Input: part model. Units: mm. Frame: model coordinates. Face numbers are marked on the shaded views. A direction names the side the tool comes from. Round coordinates to 2 decimals unless told otherwise and drop trailing zeros. Order: outer loops, then holes, each group sorted by start corner. A loop starts at its lowest first (then second) coordinate and runs counter-clockwise, first axis right, second up. Notation, with made-up numbers: M 58,66.5 L 94,66.5 A12 ccw 94,71.5 Z; hole C 74,6 d5. An arc over 180 degrees is marked long. One line per question, with ' | ' between items.
```python
from build123d import *

# Parameters (mm, degrees)
SKETCH_2_W                  = 36.9
SKETCH_2_H                  = 60.6
SKETCH_2_W_2                = 33.7
SKETCH_2_H_2                = 57.4
SKETCH_2_W_3                = 35.4
SKETCH_2_H_3                = 59.1
SKETCH_2_R                  = 3.75
SKETCH_2_R_2                = 2.25
SKETCH_2_R_3                = 0.75
EXTRUDE_1_DEPTH             = 1.5
EXTRUDE_START               = 1.5
SKETCH_2_20_W               = 36.9
SKETCH_2_20_H               = 60.6
SKETCH_2_20_W_2             = 35.4
SKETCH_2_20_H_2             = 59.1
SKETCH_2_20_W_3             = 33.7
SKETCH_2_20_H_3             = 57.4
EXTRUDE_9_DEPTH             = 12
CUT_EXTRUDE_START           = 13.5
SKETCH_2_21_W               = 35.4
SKETCH_2_21_H               = 59.1
SKETCH_2_21_W_2             = 33.7
SKETCH_2_21_H_2             = 57.4
CUT_EXTRUDE_3_DEPTH         = 1.5
EXTRUDE_START_2             = 13.5
SKETCH_2_23_R               = 3
SKETCH_2_23_R_2             = 1.6
EXTRUDE_10_DEPTH            = 10
FILLET_2_R                  = 3.5
HOLE_WIZARD_M32_D           = 3.4
HOLE_WIZARD_M32_CSINK_D     = 6.72
HOLE_WIZARD_M32_CSINK_ANGLE = 90
SKETCH_12_W                 = 1.6
SKETCH_12_H                 = 15.6
SKETCH_12_H_2               = 15.8
SKETCH_12_H_3               = 12.5
CUT_EXTRUDE_4_DEPTH         = 1.65
SKETCH_13_W                 = 3
SKETCH_13_H                 = 10
SKETCH_13_H_2               = 7
SKETCH_13_W_2               = 10
SKETCH_13_H_3               = 3
EXTRUDE_11_DEPTH            = 16.2


with BuildPart() as part:
    # Эскиз2 → Бобышка-Вытянуть1 (new body)
    # profile 1 of 15: a face of its own
    with BuildSketch(Plane(origin=(0, 0, 0), x_dir=(1, 0, 0), z_dir=(0, 1, 0))):
        with Locations((16.65, 28.5)):
            Rectangle(SKETCH_2_W, SKETCH_2_H)
        with Locations((16.65, 28.5)):
            Rectangle(SKETCH_2_W_2, SKETCH_2_H_2, mode=Mode.SUBTRACT)
    # profile 2 of 15: a face of its own
    with BuildSketch(Plane(origin=(0, 0, 0), x_dir=(1, 0, 0), z_dir=(0, 1, 0))):
        with Locations((16.65, 28.5)):
            Rectangle(SKETCH_2_W_3, SKETCH_2_H_3)
        with Locations((16.65, 28.5)):
            Rectangle(SKETCH_2_W_2, SKETCH_2_H_2, mode=Mode.SUBTRACT)
    # profile 3 of 15: a face of its own
    with BuildSketch(Plane(origin=(0, 0, 0), x_dir=(1, 0, 0), z_dir=(0, 1, 0))):
        with BuildLine():
            Line((-0.2, 57.2), (-0.2, -0.2))
            Line((-0.2, -0.2), (33.5, -0.2))
            Line((33.5, -0.2), (33.5, 10.050490243))
            ThreePointArc((33.5, 10.050490243), (27, 12.6), (33.5, 15.149509757))
            Line((33.5, 15.149509757), (33.5, 57.2))
            Line((33.5, 57.2), (-0.2, 57.2))
        make_face()
        with Locations((5.1, 19.73)):
            Circle(SKETCH_2_R, mode=Mode.SUBTRACT)
        with Locations((5.1, 41.13)):
            Circle(SKETCH_2_R, mode=Mode.SUBTRACT)
        with Locations((23.55, 45)):
            Circle(SKETCH_2_R, mode=Mode.SUBTRACT)
    # profile 4 of 15: a face of its own
    with BuildSketch(Plane(origin=(0, 0, 0), x_dir=(1, 0, 0), z_dir=(0, 1, 0))):
        with Locations((23.55, 45)):
            Circle(SKETCH_2_R)
        with Locations((23.55, 45)):
            Circle(SKETCH_2_R_2, mode=Mode.SUBTRACT)
    # profile 5 of 15: a face of its own
    with BuildSketch(Plane(origin=(0, 0, 0), x_dir=(1, 0, 0), z_dir=(0, 1, 0))):
        with Locations((23.55, 45)):
            Circle(SKETCH_2_R_2)
        with Locations((23.55, 45)):
            Circle(SKETCH_2_R_3, mode=Mode.SUBTRACT)
    # profile 6 of 15: a face of its own
    with BuildSketch(Plane(origin=(0, 0, 0), x_dir=(1, 0, 0), z_dir=(0, 1, 0))):
        with Locations((23.55, 45)):
            Circle(SKETCH_2_R_3)
    # profile 7 of 15: a face of its own
    with BuildSketch(Plane(origin=(0, 0, 0), x_dir=(1, 0, 0), z_dir=(0, 1, 0))):
        with Locations((5.1, 41.13)):
            Circle(SKETCH_2_R)
        with Locations((5.1, 41.13)):
            Circle(SKETCH_2_R_2, mode=Mode.SUBTRACT)
    # profile 8 of 15: a face of its own
    with BuildSketch(Plane(origin=(0, 0, 0), x_dir=(1, 0, 0), z_dir=(0, 1, 0))):
        with Locations((5.1, 41.13)):
            Circle(SKETCH_2_R_2)
        with Locations((5.1, 41.13)):
            Circle(SKETCH_2_R_3, mode=Mode.SUBTRACT)
    # profile 9 of 15: a face of its own
    with BuildSketch(Plane(origin=(0, 0, 0), x_dir=(1, 0, 0), z_dir=(0, 1, 0))):
        with Locations((5.1, 41.13)):
            Circle(SKETCH_2_R_3)
    # profile 10 of 15: a face of its own
    with BuildSketch(Plane(origin=(0, 0, 0), x_dir=(1, 0, 0), z_dir=(0, 1, 0))):
        with Locations((5.1, 19.73)):
            Circle(SKETCH_2_R)
        with Locations((5.1, 19.73)):
            Circle(SKETCH_2_R_2, mode=Mode.SUBTRACT)
    # profile 11 of 15: a face of its own
    with BuildSketch(Plane(origin=(0, 0, 0), x_dir=(1, 0, 0), z_dir=(0, 1, 0))):
        with Locations((5.1, 19.73)):
            Circle(SKETCH_2_R_2)
        with Locations((5.1, 19.73)):
            Circle(SKETCH_2_R_3, mode=Mode.SUBTRACT)
    # profile 12 of 15: a face of its own
    with BuildSketch(Plane(origin=(0, 0, 0), x_dir=(1, 0, 0), z_dir=(0, 1, 0))):
        with Locations((5.1, 19.73)):
            Circle(SKETCH_2_R_3)
    # profile 13 of 15: a face of its own
    with BuildSketch(Plane(origin=(0, 0, 0), x_dir=(1, 0, 0), z_dir=(0, 1, 0))):
        with BuildLine():
            ThreePointArc((33.5, 15.149509757), (27, 12.6), (33.5, 10.050490243))
            Line((33.5, 10.050490243), (33.5, 15.149509757))
        make_face()
        with Locations((30.75, 12.6)):
            Circle(SKETCH_2_R_2, mode=Mode.SUBTRACT)
    # profile 14 of 15: a face of its own
    with BuildSketch(Plane(origin=(0, 0, 0), x_dir=(1, 0, 0), z_dir=(0, 1, 0))):
        with Locations((30.75, 12.6)):
            Circle(SKETCH_2_R_2)
        with Locations((30.75, 12.6)):
            Circle(SKETCH_2_R_3, mode=Mode.SUBTRACT)
    # profile 15 of 15: a face of its own
    with BuildSketch(Plane(origin=(0, 0, 0), x_dir=(1, 0, 0), z_dir=(0, 1, 0))):
        with Locations((30.75, 12.6)):
            Circle(SKETCH_2_R_3)
    extrude(amount=EXTRUDE_1_DEPTH)

    # Эскиз2<20> → Бобышка-Вытянуть9 (add)
    # profile 1 of 2: a face of its own
    with BuildSketch(Plane(origin=(0, 0, 0), x_dir=(1, 0, 0), z_dir=(0, 1, 0)).offset(EXTRUDE_START)):
        with Locations((16.65, 28.5)):
            Rectangle(SKETCH_2_20_W, SKETCH_2_20_H)
        with Locations((16.65, 28.5)):
            Rectangle(SKETCH_2_20_W_2, SKETCH_2_20_H_2, mode=Mode.SUBTRACT)
    # profile 2 of 2: a face of its own
    with BuildSketch(Plane(origin=(0, 0, 0), x_dir=(1, 0, 0), z_dir=(0, 1, 0)).offset(EXTRUDE_START)):
        with Locations((16.65, 28.5)):
            Rectangle(SKETCH_2_20_W_2, SKETCH_2_20_H_2)
        with Locations((16.65, 28.5)):
            Rectangle(SKETCH_2_20_W_3, SKETCH_2_20_H_3, mode=Mode.SUBTRACT)
    extrude(amount=EXTRUDE_9_DEPTH)

    # Эскиз2<21> → Вырез-Вытянуть3 (cut)
    with BuildSketch(Plane(origin=(0, 0, 0), x_dir=(1, 0, 0), z_dir=(0, 1, 0)).offset(CUT_EXTRUDE_START)):
        with Locations((16.65, 28.5)):
            Rectangle(SKETCH_2_21_W, SKETCH_2_21_H)
        with Locations((16.65, 28.5)):
            Rectangle(SKETCH_2_21_W_2, SKETCH_2_21_H_2, mode=Mode.SUBTRACT)
    extrude(amount=-CUT_EXTRUDE_3_DEPTH, mode=Mode.SUBTRACT)

    # Эскиз2<23> → Бобышка-Вытянуть10 (add)
    # profile 1 of 4: a face of its own
    with BuildSketch(Plane(origin=(0, 0, 0), x_dir=(1, 0, 0), z_dir=(0, 1, 0)).offset(EXTRUDE_START_2)):
        with BuildLine():
            ThreePointArc((7.877165354, 60.877946056), (6.171513422, 59.351502874), (3.95, 58.8))
            Line((3.95, 58.8), (29.35, 58.8))
            ThreePointArc((29.35, 58.8), (27.128486578, 59.351502874), (25.422834646, 60.877946056))
            Line((25.422834646, 60.877946056), (21.403937008, 66.784591616))
            ThreePointArc((21.403937008, 66.784591616), (19.339200458, 68.632391258), (16.65, 69.3))
            ThreePointArc((16.65, 69.3), (13.960799542, 68.632391258), (11.896062992, 66.784591616))
            Line((11.896062992, 66.784591616), (7.877165354, 60.877946056))
        make_face()
        with Locations((16.65, 63.55)):
            Circle(SKETCH_2_23_R, mode=Mode.SUBTRACT)
    # profile 2 of 4: a face of its own
    with BuildSketch(Plane(origin=(0, 0, 0), x_dir=(1, 0, 0), z_dir=(0, 1, 0)).offset(EXTRUDE_START_2)):
        with Locations((16.65, 63.55)):
            Circle(SKETCH_2_23_R)
        with Locations(Location((16.65, 63.55, 0), (0, 0, 90))):
            Circle(SKETCH_2_23_R_2, mode=Mode.SUBTRACT)
    # profile 3 of 4: a face of its own
    with BuildSketch(Plane(origin=(0, 0, 0), x_dir=(1, 0, 0), z_dir=(0, 1, 0)).offset(EXTRUDE_START_2)):
        with BuildLine():
            Line((29.35, -1.8), (3.95, -1.8))
            ThreePointArc((3.95, -1.8), (6.171513422, -2.351502874), (7.877165354, -3.877946056))
            Line((7.877165354, -3.877946056), (11.896062992, -9.784591616))
            ThreePointArc((11.896062992, -9.784591616), (13.960799542, -11.632391258), (16.65, -12.3))
            ThreePointArc((16.65, -12.3), (19.339200458, -11.632391258), (21.403937008, -9.784591616))
            Line((21.403937008, -9.784591616), (25.422834646, -3.877946056))
            ThreePointArc((25.422834646, -3.877946056), (27.128486578, -2.351502874), (29.35, -1.8))
        make_face()
        with Locations((16.65, -6.55)):
            Circle(SKETCH_2_23_R, mode=Mode.SUBTRACT)
    # profile 4 of 4: a face of its own
    with BuildSketch(Plane(origin=(0, 0, 0), x_dir=(1, 0, 0), z_dir=(0, 1, 0)).offset(EXTRUDE_START_2)):
        with Locations((16.65, -6.55)):
            Circle(SKETCH_2_23_R)
        with Locations(Location((16.65, -6.55, 0), (0, 0, 90))):
            Circle(SKETCH_2_23_R_2, mode=Mode.SUBTRACT)
    extrude(amount=-EXTRUDE_10_DEPTH)

    # Скругление2
    fillet_2_edges = [part.edges().sort_by_distance(p)[0] for p in [
        (16.65, 1.5, -57.2),
        (-0.2, 1.5, -28.5),
        (33.5, 1.5, -28.5),
        (16.65, 1.5, 0.2),
        (16.65, 0, -58.8),
        (35.1, 0, -28.5),
        (16.65, 0, 1.8),
        (-1.8, 0, -28.5),
    ]]
    fillet(fillet_2_edges, radius=FILLET_2_R - 0.0001)  # a hair under: the kernel refuses the full size

    # Зенковка для  винта с потайной головкой с внутренним шестигранником M32 (through all)
    with Locations(Plane(origin=(0, 3.5, 0), x_dir=(-1, 0, 0), z_dir=(0, -1, 0))):
        with Locations((-16.65, 63.55), (-16.65, -6.55)):
            CounterSinkHole(HOLE_WIZARD_M32_D / 2, HOLE_WIZARD_M32_CSINK_D / 2, counter_sink_angle=HOLE_WIZARD_M32_CSINK_ANGLE)

    # Эскиз12 → Вырез-Вытянуть4 (cut)
    with BuildSketch(Plane(origin=(0, 13.5, 0), x_dir=(1, 0, 0), z_dir=(0, 1, 0))):
        with Locations((-1, 48)):
            Rectangle(SKETCH_12_W, SKETCH_12_H)
        with Locations((-1, 26.6)):
            Rectangle(SKETCH_12_W, SKETCH_12_H_2)
        with Locations((-1, 7.05)):
            Rectangle(SKETCH_12_W, SKETCH_12_H_3)
    extrude(amount=-CUT_EXTRUDE_4_DEPTH, mode=Mode.SUBTRACT)

    # Эскиз13 → Бобышка-Вытянуть11 (add)
    with BuildSketch(Plane(origin=(0, 1.5, 0), x_dir=(1, 0, 0), z_dir=(0, 1, 0))):
        with Locations((10.3, 44.2)):
            Rectangle(SKETCH_13_W, SKETCH_13_H)
        with Locations((24, 42.7)):
            Rectangle(SKETCH_13_W, SKETCH_13_H_2)
        with Locations((16.65, 6.8)):
            Rectangle(SKETCH_13_W_2, SKETCH_13_H_3)
    extrude(amount=EXTRUDE_11_DEPTH)


solid = part.part
```
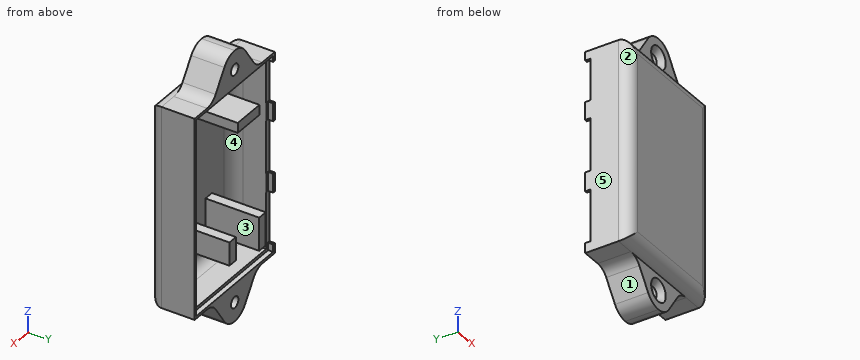
Item 1: Section query A-A, the plane y = 15.25. Return loops of the section in (x, z).
Report:
outline: M 8.8,-49.2 L 11.8,-49.2 L 11.8,-39.2 L 8.8,-39.2 Z; M 11.65,-8.3 L 21.65,-8.3 L 21.65,-5.3 L 11.65,-5.3 Z; M 22.5,-46.2 L 25.5,-46.2 L 25.5,-39.2 L 22.5,-39.2 Z
Item 2: Line query: line 1 along Z through (x, y) = (16.65, 8.5); line 2 along X through (y, z) = (11.25, -47.5); line 3 along Z through (x, y) = (20.5, 9.5). Output: solid intervals per line, ascending. Write a range as from..to.
Report:
line 1: -69.3..-65.25, -61.85..-57.2, -8.3..-5.3, 0.2..4.85, 8.25..12.3 | line 2: -1.8..-0.2, 8.8..11.8, 33.5..35.1 | line 3: -67.82..-57.2, -8.3..-5.3, 0.2..10.82
Item 3: Section query C-C, the plane z = -63.55. Return loops of the section in (x, y).
Report:
outline: M 9.7,3.5 L 13.29,3.5 L 14.95,5.16 L 14.95,13.5 L 9.7,13.5 Z; M 18.35,5.16 L 20.01,3.5 L 23.6,3.5 L 23.6,13.5 L 18.35,13.5 Z
Item 4: Access query for the marked faces 4 and 5. Directions: +Z, -Z, +X, -X, +Y, -Y. A direction counts if a zero-diameter tool reaches every point of the face in a straight line with its end or side. Return the directions, or none.
Report:
face 4: +Y | face 5: +Z, -Z, -X, +Y, -Y
Item 5: Mould query, pull axis Z, two halves, no side actions, for the marked faces 1, 2 and 3. Classes: +Z half, -Z half, draft (parallel to the pull), parting line (faces both ways), or undercut.
Report:
face 1: -Z half | face 2: draft | face 3: undercut
Item 6: Section query B-B, the plane z = -42.5. Return loops of the section in (x, y).
Report:
outline: M -1.8,3.5 A3.5 ccw 1.7,0 L 31.6,0 A3.5 ccw 35.1,3.5 L 35.1,13.5 L 34.35,13.5 L 34.35,12 L 33.5,12 L 33.5,5 A3.5 cw 30,1.5 L 25.5,1.5 L 25.5,17.7 L 22.5,17.7 L 22.5,1.5 L 11.8,1.5 L 11.8,17.7 L 8.8,17.7 L 8.8,1.5 L 3.3,1.5 A3.5 cw -0.2,5 L -0.2,11.85 L -1.8,11.85 Z
Item 7: First-contact query: pin 1 (0.5 mm diameter, centred on x = -1.5, y = 12.5, fed in from -Z); pin 2 (2 mm diameter, centred on x = 12.5, z = -50.5, fed in from +Y); pin 3 (0.6 mm diameter, centred on x = -1.5, z = -16, fed in from +Y). Flat tips, straight axial feed; report the tip coordinate or a pass-through.
Report:
pin 1: z = -58.8 | pin 2: y = 1.5 | pin 3: y = 13.5
Item 8: Section query D-D, the plane y = 9. Give the number of separate pieces and of enclosed holes in the cut face, plus the area to 3 significant figures.
Report:
separate pieces: 4 | enclosed holes: 3 | area: 641 mm²
